Part model, mm, in its own coordinate system. A direction names the side the tool comes from. Coordinates: 2 decimals unless noted, no trailing zeros. Order: outer loops, then holes, each group sorted by start corner. A loop starts at its lowest first (then second) coordinate and runs counter-clockwise, first axis right, second up.
1) Cut at B-B (z = 0). List the corners of the cut face in (x, y).
2) Tool access for faces 4 (the flat face through (-35.094, -8, 1)), 5 (the flat face through (-40.576, 0, 18)), 6 (the cylindrical face through (-134, 8, -6)), 7 (the flat face through (-35.094, 7, 0)), 8 (the flat face through (-16, 0, 20)): list every direction of +Z, -Z, +X, -X, +Y, -Y with a clear straight run to the whole face (end or side of a thin tool).
3) Pin check, flat tips, straight feed: pin 1 Ø10 at (x, y) = (-93, -3.5) entering from +Z; pin 2 Ø4 at (x, y) = (-61.5, 7) entering from -Z; pin 3 Ø1.4 at (y, z) = (-7.5, -2.5) entering from +X. Stop position of each tip, or through.
4) Mould opens along Z. For faces 1 (the flat face through (-24.798, 0, 0)), 2 (the flat face through (-21, 0, 15)), 3 (the flat face through (-30, 0, -15)) say: +Z half, -Z half, draft (parallel to the pull), parting line (faces both ways), or undercut.
5) Cut at D-D (x = -18.5). List the corners of the cut face in (y, z), and give its area (3 significant figures).
6) Wall check: L1, parallel to X at y = -0.5, z = 2.5; L2, parallel to X at y = 1, z = 5; L3, parallel to Z at x = -40.5, y = -7.75. Give the ranges that are in metal, low to high.
7) Cut at C-C (y = 3). List the corners of the cut face in (x, z).
8) Cut at A-A (y = -8). List the corners of the cut face in (x, z).
```python
from build123d import *

# Parameters (mm, degrees)
SZKIC1_R                    = 10
DODANIE_WYCI_GNI_CIE1_DEPTH = 15
DODANIE_WYCI_GNI_CIE2_START = 5
DODANIE_WYCI_GNI_CIE2_DEPTH = 5
SZKIC3_W                    = 10.29571442
SZKIC3_H                    = 10.783406156
DODANIE_WYCI_GNI_CIE3_DEPTH = 30
SZKIC4_R                    = 10
DODANIE_WYCI_GNI_CIE4_DEPTH = 200


with BuildPart() as part:
    # Szkic1 → Dodanie-wyciągnięcie1 (new, symmetric)
    with BuildSketch(Plane.XY):
        Circle(SZKIC1_R)
    extrude(amount=DODANIE_WYCI_GNI_CIE1_DEPTH, both=True)

    # Szkic2 → Dodanie-wyciągnięcie2 (add)
    with BuildSketch(Plane.XY.offset(15).offset(DODANIE_WYCI_GNI_CIE2_START)):
        with BuildLine():
            Line((0, 10), (-40.57595794, 10))
            Line((-40.57595794, 10), (-40.57595794, -10))
            Line((-40.57595794, -10), (0, -10))
            ThreePointArc((0, -10), (10, 0), (0, 10))
        make_face()
    extrude(amount=-DODANIE_WYCI_GNI_CIE2_DEPTH)

    # Szkic3 → Dodanie-wyciągnięcie3 (add)
    with BuildSketch(Plane(origin=(0, 0, 15), x_dir=(-1, 0, 0), z_dir=(0, 0, -1))):
        with Locations((29.945825027, 0)):
            Rectangle(SZKIC3_W, SZKIC3_H)
    extrude(amount=DODANIE_WYCI_GNI_CIE3_DEPTH)

    # Szkic4 → Dodanie-wyciągnięcie4 (add)
    with BuildSketch(Plane.ZY.offset(35.093682237)):
        with Locations(Location((0, 0, 0), (0, 0, 147.37282405))):
            Circle(SZKIC4_R)
    extrude(amount=DODANIE_WYCI_GNI_CIE4_DEPTH)


solid = part.part
```
Geometry check:
1. outline: (-235.09, -10) - (-35.09, -10) - (-35.09, -5.39) - (-24.8, -5.39) - (-24.8, 5.39) - (-35.09, 5.39) - (-35.09, 10) - (-235.09, 10) - close; circle Ø20 at (0, 0)
2. face 4: -Z, -Y
2. face 5: +Z, -X, +Y, -Y
2. face 6: -X
2. face 7: -Z, +Y
2. face 8: +Z, +X, -X, +Y, -Y
3. pin 1: stops at z = 10
3. pin 2: stops at z = -8.66
3. pin 3: stops at x = 7.33
4. face 1: draft
4. face 2: undercut
4. face 3: -Z half
5. outline: (-10, 15) - (10, 15) - (10, 20) - (-10, 20) - close
5. area: 100 mm2
6. L1: x = -235.09 to -24.8, -9.99 to 9.99
6. L2: x = -235.09 to -24.8, -9.95 to 9.95
6. L3: z = -6.32 to 6.32, 15 to 20
7. outline: (-235.09, -9.54) - (-35.09, -9.54) - (-35.09, -15) - (-24.8, -15) - (-24.8, 15) - (-9.54, 15) - (-9.54, -15) - (9.54, -15) - (9.54, 20) - (-40.58, 20) - (-40.58, 15) - (-35.09, 15) - (-35.09, 9.54) - (-235.09, 9.54) - close
8. outline: (-235.09, -6) - (-35.09, -6) - (-35.09, 6) - (-235.09, 6) - close; (-40.58, 15) - (-6, 15) - (-6, -15) - (6, -15) - (6, 20) - (-40.58, 20) - close
